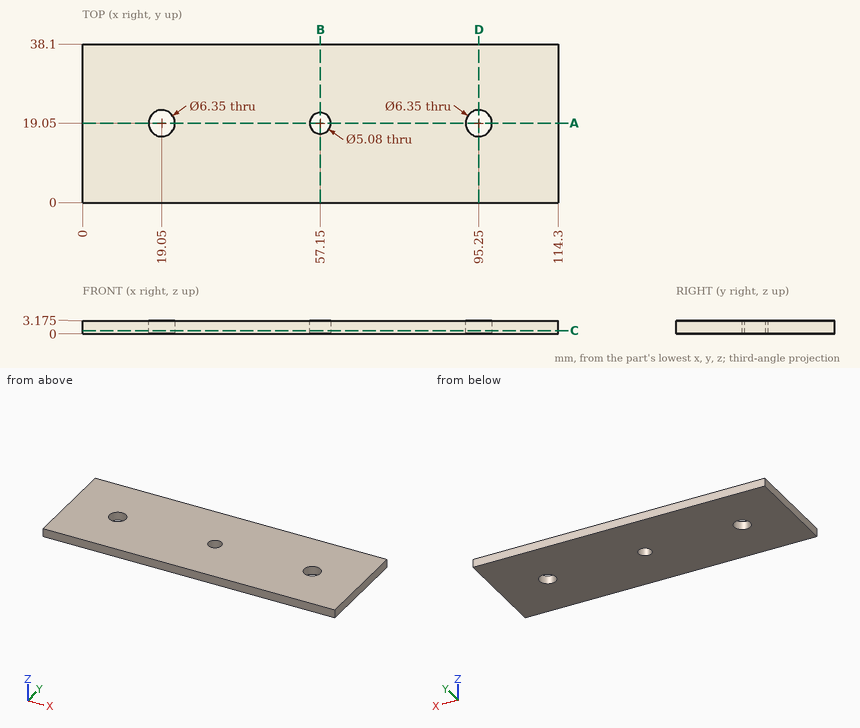
Geometry check sheet. Reference: drawing and pictorial views, mm from the part's lowest x, y, z. Coordinates: 2 decimals unless noted, no trailing zeros. Order: outer loops, then holes, each group sorted by start corner. A loop starts at its lowest first (then second) coordinate and runs counter-clockwise, first axis right, second up. Notation, with made-up numbers: M 58.25,57.25 L 64.25,57.25 A24 cw 64.25,69.25 Z; hole C -4.75,69 d8. An arc over 180 degrees is marked long. Write each question's results on one line, items separated by ' | '. Start each with the question number.
1. Cross-section at D-D on x = 95.25. Record the cut outline in (y, z) (3 decimals), and give its area (3 significant figures).
2. Cross-section at A-A on y = 19.05. Record the cut outline in (x, z) (3 decimals), and give its area (3 significant figures).
3. Material ranges on probe 1 along Y at (x, z) = (95.25, 1.9) (3 decimals); probe 2 along Y at (x, z) = (57.15, 1.7); probe 3 along X at (y, z) = (18.5, 1.2), recorded low to high.
4. Cross-section at B-B on x = 57.15. Record the cut outline in (y, z) (3 decimals), and give its area (3 significant figures).
5. Cross-section at C-C on z = 0.75. Record the cut outline in (x, y) (3 decimals), and give its area (3 significant figures).
Checks:
1) outline: M 0,0 L 15.875,0 L 15.875,3.175 L 0,3.175 Z; M 22.225,0 L 38.1,0 L 38.1,3.175 L 22.225,3.175 Z | area: 101 mm²
2) outline: M 0,0 L 15.875,0 L 15.875,3.175 L 0,3.175 Z; M 22.225,0 L 54.61,0 L 54.61,3.175 L 22.225,3.175 Z; M 59.69,0 L 92.075,0 L 92.075,3.175 L 59.69,3.175 Z; M 98.425,0 L 114.3,0 L 114.3,3.175 L 98.425,3.175 Z | area: 306 mm²
3) probe 1: y = 0 to 15.875, 22.225 to 38.1 | probe 2: y = 0 to 16.51, 21.59 to 38.1 | probe 3: x = 0 to 15.92, 22.18 to 54.67, 59.63 to 92.12, 98.38 to 114.3
4) outline: M 0,0 L 16.51,0 L 16.51,3.175 L 0,3.175 Z; M 21.59,0 L 38.1,0 L 38.1,3.175 L 21.59,3.175 Z | area: 105 mm²
5) outline: M 0,0 L 114.3,0 L 114.3,38.1 L 0,38.1 Z; hole C 19.05,19.05 d6.35; hole C 57.15,19.05 d5.08; hole C 95.25,19.05 d6.35 | area: 4,270 mm²
